Geometry: final body of the model. Coordinates: model frame, mm. Give positions to 0.01 mm unless a question says otherwise; leave off trailing zeros. Loops run counter-clockwise (first coordinate to the right, second up) from the corner with the lowest first, then second, coordinate; pieces in that order, holes last. Notation, with made-up numbers: (-24, 77) - (23, 77) arc R32 cw to (23, 114) - close; hole circle Ø3 at (-16, -36.75). An arc over 180 degrees is marked (long way). Use one line per item in the form item = value.
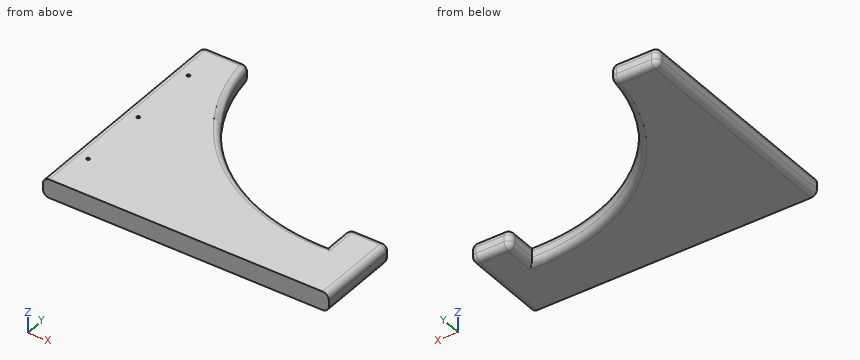
```python
from build123d import *

# Parameters (mm, degrees)
F1_DEPTH = 6
F3_D     = 1
F3_DEPTH = 1
F3_TIP   = 0.3004303095
F4_R     = 2


with BuildPart() as f1:
    # F0 (on Top) → F1 (new body)
    with BuildSketch(Plane.XY):
        with BuildLine():
            Line((-43.1737847788, 64.6250816927), (-43.1737847788, -8.3749183073))
            Line((-43.1737847788, -8.3749183073), (48.8262152212, -8.3749183073))
            Line((48.8262152212, -8.3749183073), (48.8262152212, 19.6250816927))
            Line((48.8262152212, 19.6250816927), (35.8262152212, 19.6250816927))
            Line((35.8262152212, 19.6250816927), (35.8262152212, 9.6250816927))
            ThreePointArc((35.8262152212, 9.6250816927), (-6.8545907303, 24.6965074946), (-28.1737847788, 64.6250816927))
            Line((-28.1737847788, 64.6250816927), (-43.1737847788, 64.6250816927))
        make_face()
    extrude(amount=F1_DEPTH)

    # F3
    with Locations(Plane.XY.offset(6)):
        with Locations((-38.1737847788, 51.1250816927), (-38.1737847788, 28.1250816927), (-38.1737847788, 5.1250816927)):
            Hole(F3_D / 2, depth=F3_DEPTH)
            with Locations((0, 0, -(F3_DEPTH + F3_TIP / 2))):  # 118° drill point
                Cone(0, F3_D / 2, F3_TIP, mode=Mode.SUBTRACT)

    # F4
    f4_edges = [f1.edges().sort_by_distance(p)[0] for p in [
        (48.826215, 19.625082, 3),
        (48.826215, 5.625082, 0),
        (48.826215, 5.625082, 6),
        (42.326215, 19.625082, 6),
        (42.326215, 19.625082, 0),
        (35.826215, 14.625082, 6),
        (-6.854591, 24.696507, 6),
        (35.826215, 14.625082, 0),
        (-6.854591, 24.696507, 0),
        (-35.673785, 64.625082, 0),
        (-35.673785, 64.625082, 6),
        (-43.173785, 28.125082, 0),
        (-43.173785, 28.125082, 6),
        (35.826215, 19.625082, 3),
        (-28.173785, 64.625082, 3),
        (-43.173785, 64.625082, 3),
    ]]
    fillet(f4_edges, radius=F4_R)


solid = f1.part
```
(1) Material intervals for L1, parallel to X at y = 3.5, z = 1.5; L2, parallel to X at y = 60.5, z = 3.25; L3, parallel to Y at x = -5, z = 3.75, sorted ascending. Write a range as from..to.
Solution:
L1 = -43.11..48.76
L2 = -43.17..-27.54
L3 = -8.37..23.16
(2) Cut plane A-A (z = 1). Return the cut outline in (x, y), plus the area to 3 significant figures.
Solution:
outline = (-42.91, -8.37) - (48.56, -8.37) - (48.56, 17.63) arc R1.73 ccw to (46.83, 19.36) - (37.83, 19.36) arc R1.73 ccw to (36.09, 17.63) - (36.09, 9.37) arc R62.78 cw to (-28.21, 62.88) arc R1.73 ccw to (-29.92, 64.36) - (-41.17, 64.36) arc R1.73 ccw to (-42.91, 62.63) - close
area = 3,360 mm2
(3) Pin query (flat end, axial travel): P1, Ø6, axis at x = -12.5, y = 33.5, coming from the +Z side; P2, Ø2, axis at x = 44, z = 2.5, coming from the +Y side; P3, Ø1.5, axis at x = 11, y = 14.5, coming from the -Z side; P4, Ø12, axis at x = -8.5, y = 37.5, coming from the +Z side. Return the tip coordinate at first contact, or that it passes through.
Solution:
P1 = 5.63
P2 = 19.63
P3 = 1.08
P4 = through
